Autodesk Inventor part; units mm, degrees
ref_plane "YZ Plane" through (0, 0, 0) normal (1, 0, 0) x (0, 1, 0)
ref_plane "XZ Plane" through (0, 0, 0) normal (0, 1, 0) x (-1, 0, 0)
ref_plane "XY Plane" through (0, 0, 0) normal (0, 0, 1) x (1, 0, 0)
sketch "Sketch1" plane through (0, 0, 0) normal (0, 1, 0) x (-1, 0, 0)
  line L0 (300, 0) -> (-300, 0)
  line L1 (-300, 0) -> (-300, 600)
  line L2 (-300, 600) -> (300, 600)
  line L3 (300, 600) -> (300, 0)
  point P0 (0, 0)
  point P1 (0, 0)
  dimension "d0" = 600
  dimension "d1" = 600
extrude "Extrusion1" add sketch "Sketch1" along normal blind 850
sketch "Sketch3" plane through (-300, 0, 600) normal (0, 0, 1) x (1, 0, 0)
  line L0 (0, 0) -> (600, 0)
  line L1 (600, 0) -> (600, 850)
  line L2 (0, 0) -> (600, 0)
  line L3 (600, 0) -> (600, 120)
  line L4 (600, 120) -> (0, 120)
  line L5 (0, 120) -> (0, 0)
  point P0 (300, 0)
  dimension "d9" = 120
extrude "Extrusion3" cut sketch "Sketch3" against normal blind 20
properties part number "Mobile lavastoviglie"
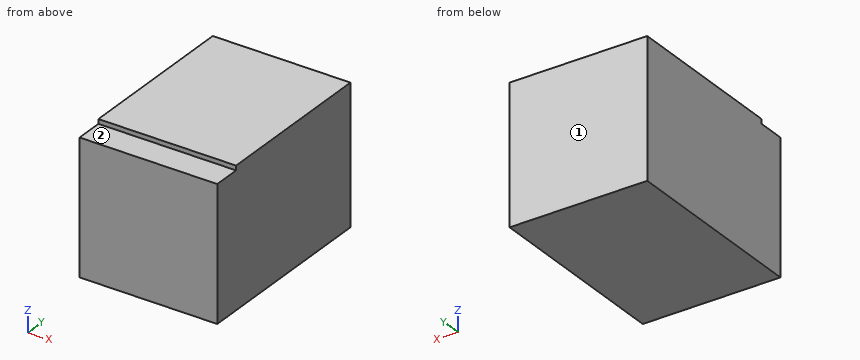
Could you check a few things on this model? Use its own coordinates, in mm. Face numbers are marked on the shaded views. A direction names the side the tool comes from. Round coordinates to 2 decimals unless told otherwise and drop trailing zeros. Write each loop counter-clockwise with the first axis right and the second up, starting at its lowest first coordinate (ties: lowest second). Pieces come first, ordered by that corner, then holes.
(1) Which directions (+Z, -Z, +X, -X, +Y, -Y) give clear straight access to the entire face, cutting with the end or side of a thin tool? Please do the marked faces 1 and 2.
Findings below:
face 1: +Z, -Z, +X, -X, +Y
face 2: +Z, +X, -X, -Y
(2) For pin 1 (6 mm diameter, centred on x = -8, z = 585.5, fed in from -Y), with a flat end and sliding along its axis, tell me the tip position at first contact or that it passes through.
Findings below:
pin 1: stops at y = 120
(3) If I drill on probe 1 along Z at (x, y) = (3.5, 87), over which ranges is the centre line in solid material (lowest first)?
Findings below:
probe 1: z = 0 to 580
(4) Suppose I cut it at A-A on y = 97. Write out the boundary of the cut face in (x, z), and give its area (3 significant figures).
Findings below:
outline: (-300, 0) - (300, 0) - (300, 580) - (-300, 580) - close
area: 348,000 mm2
